Design review of the part built by this model. Coordinates are the model's own, in mm. Face numbers are marked on the shaded views. A direction names the side the tool comes from. Round coordinates to 2 decimals unless told otherwise and drop trailing zeros. Loops run counter-clockwise (first coordinate to the right, second up) from the corner with the lowest first, then second, coordinate; pieces in that order, holes last. Notation, with made-up numbers: (-20.5, 24.5) - (23.5, 24.5) arc R25 ccw to (23.5, 58.5) - close; hole circle Ø5 at (66, 65). An arc over 180 degrees is marked (long way). Return JSON: item names as keys, results as strings. Group by question number.
(1) Wall thickness on L1, parallel to Y at x = 0, z = -31 (1 decimal); L2, parallel to Z at x = 1, y = -0.5; L3, parallel to Z at x = 2, y = 1.25: over which ranges is each line inside the solid? List them lowest first. Write a range as [from, to].
(2) We need section D-D, the plane z = -4. Write out the cut boundary in (x, y) (1 decimal).
(3) The part is to be moulded in two halves that separate along Y. For the marked faces 1 and 2, say which applies: pulls with the +Y half, pulls with the -Y half, needs draft (parallel to the pull), parting line crosses it, or undercut.
(4) Clearance check with flat-ended pins moving along their axes: pin 1 (3 mm diameter, centred on x = -2, z = -17, fed in from +Y); pin 2 (1 mm diameter, centred on x = 0, y = 0.5, fed in from -Z); pin 3 (1.5 mm diameter, centred on y = -1, z = -20.5, fed in from -X). State where each tip first meets the part, or that it passes through.
(5) For the marked faces 3 and 4, list the 3-axis set-ups (+Z, -Z, +X, -X, +Y, -Y) from which the entire face can be reached by the end or side of a thin tool; tool diameter is ignored.
from build123d import *

# Parameters (mm, degrees)
CHAMFER1_SIZE = 0.254


with BuildPart() as part:
    # Sketch1 → Revolve1 (revolve)
    with BuildSketch(Plane(origin=(0, 0, 0), x_dir=(0, 0, -1), z_dir=(1, 0, 0)), mode=Mode.PRIVATE) as revolve1_sk:
        Polygon((0, 0), (0, 1.5875), (10.16, 1.5875), (10.16, 3.175), (16.9545, 3.175), (16.9545, 2.921), (17.6911, 2.921), (17.6911, 3.175), (32.7914, 3.175), (32.7914, 1.5875), (26.4414, 1.5875), (26.4414, 0), align=None)
    revolve(revolve1_sk.sketch.rotate(Axis((0, 0, -26.4414), (0, 0, 1)), 90), axis=Axis((0, 0, -26.4414), (0, 0, 1)))

    # Chamfer1
    chamfer1_edges = [part.edges().sort_by_distance(p)[0] for p in [
        (3.175, 0, -10.16),
        (1.5875, 0, 0),
        (3.175, 0, -32.7914),
    ]]
    chamfer(chamfer1_edges, length=CHAMFER1_SIZE)


solid = part.part
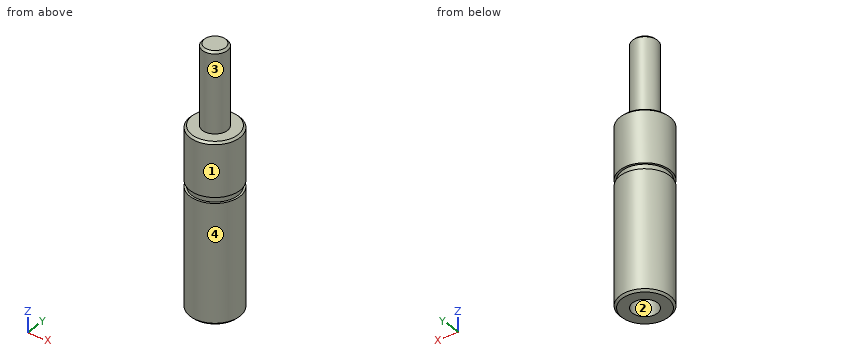
Solutions:
{
 "1": {"L1": "[-3.2, -1.6], [1.6, 3.2]", "L2": "[-26.44, 0]", "L3": "[-32.79, -10.16]"},
 "2": {"outline": "circle Ø3.2 at (0, 0)"},
 "3": {"face 1": "parting line crosses it", "face 2": "undercut"},
 "4": {"pin 1": "y = 3.14", "pin 2": "z = -26.44", "pin 3": "x = -3.17"},
 "5": {"face 3": "+Z", "face 4": "+Z, -Z"}
}
